from build123d import *

# Parameters (mm, degrees)
SALIENTE_EXTRUIR1_DEPTH = 6
CROQUIS2_W              = 10
CROQUIS2_H              = 6
CROQUIS2_W_2            = 6
CROQUIS2_H_2            = 10
CORTAR_EXTRUIR1_DEPTH   = 10


with BuildPart() as part:
    # Croquis1 → Saliente-Extruir1 (new body)
    with BuildSketch(Plane.XY):
        with BuildLine():
            ThreePointArc((40.600971411, -36.999917491), (17.069259083, -64.251458669), (-0.057755376, -95.922476295))
            ThreePointArc((-0.057755376, -95.922476295), (122.116838757, -322.352188967), (320.78926855, -158.870349387))
            ThreePointArc((320.78926855, -158.870349387), (317.672636714, -126.79639101), (308.439349644, -95.922476295))
            ThreePointArc((308.439349644, -95.922476295), (291.312335185, -64.251458669), (267.780622857, -36.999917491))
            ThreePointArc((267.780622857, -36.999917491), (154.190797134, 7.728122029), (40.600971411, -36.999917491))
        make_face()
        with BuildLine():
            ThreePointArc((50.939396199, -50.062499464), (51.321581101, -49.701102835), (51.705030941, -49.341048614))
            ThreePointArc((51.705030941, -49.341048614), (213.886421224, -21.26063874), (304.190797134, -158.870349387))
            ThreePointArc((304.190797134, -158.870349387), (94.978087942, -296.688545102), (50.939396199, -50.062499464))
        make_face(mode=Mode.SUBTRACT)
    extrude(amount=SALIENTE_EXTRUIR1_DEPTH)

    # Croquis2 → Cortar-Extruir1 (cut)
    with BuildSketch(Plane.XY.offset(6)):
        Polygon((139.190797134, -3.571113679), (149.190797134, -3.571113679), (149.190797134, -0.571113679), (149.190797134, 2.428886321), (139.190797134, 2.428886321), align=None)
        with Locations((164.190797134, -0.571113679)):
            Rectangle(CROQUIS2_W, CROQUIS2_H)
        with Locations((312.490032842, -148.870349387)):
            Rectangle(CROQUIS2_W_2, CROQUIS2_H_2)
        Polygon((312.490032842, -163.870349387), (315.490032842, -163.870349387), (315.490032842, -173.870349387), (309.490032842, -173.870349387), (309.490032842, -163.870349387), align=None)
        with Locations((164.190797134, -317.169585095)):
            Rectangle(CROQUIS2_W, CROQUIS2_H)
        Polygon((149.190797134, -317.169585095), (149.190797134, -314.169585095), (139.190797134, -314.169585095), (139.190797134, -320.169585095), (149.190797134, -320.169585095), align=None)
        with Locations((-4.108438574, -148.870349387)):
            Rectangle(CROQUIS2_W_2, CROQUIS2_H_2)
        Polygon((-7.108438574, -173.870349387), (-7.108438574, -163.870349387), (-4.108438574, -163.870349387), (-1.108438574, -163.870349387), (-1.108438574, -173.870349387), align=None)
        with BuildLine():
            ThreePointArc((40.806765207, -45.48631746), (40.806765207, -48.385455263), (43.705903009, -48.385455263))
            Line((43.705903009, -48.385455263), (40.806765207, -45.48631746))
        make_face()
        with BuildLine():
            Line((40.806765207, -45.48631746), (43.705903009, -48.385455263))
            ThreePointArc((43.705903009, -48.385455263), (44.15028715, -47.720387398), (44.306334108, -46.935886361))
            ThreePointArc((44.306334108, -46.935886361), (43.040835144, -45.04193332), (40.806765207, -45.48631746))
        make_face()
        with BuildLine():
            ThreePointArc((267.574829061, -45.48631746), (264.675691258, -45.48631746), (264.675691258, -48.385455263))
            Line((264.675691258, -48.385455263), (267.574829061, -45.48631746))
        make_face()
        with BuildLine():
            Line((267.574829061, -45.48631746), (264.675691258, -48.385455263))
            ThreePointArc((264.675691258, -48.385455263), (266.909761196, -48.829839403), (268.17526016, -46.935886361))
            ThreePointArc((268.17526016, -46.935886361), (268.019213202, -46.151385325), (267.574829061, -45.48631746))
        make_face()
        with BuildLine():
            ThreePointArc((268.17526016, -270.804812413), (266.909761196, -268.910859371), (264.675691258, -269.355243512))
            Line((264.675691258, -269.355243512), (267.574829061, -272.254381314))
            ThreePointArc((267.574829061, -272.254381314), (268.019213202, -271.589313449), (268.17526016, -270.804812413))
        make_face()
        with BuildLine():
            Line((267.574829061, -272.254381314), (264.675691258, -269.355243512))
            ThreePointArc((264.675691258, -269.355243512), (264.675691258, -272.254381314), (267.574829061, -272.254381314))
        make_face()
        with BuildLine():
            ThreePointArc((44.306334108, -270.804812413), (44.15028715, -270.020311377), (43.705903009, -269.355243512))
            Line((43.705903009, -269.355243512), (40.806765207, -272.254381314))
            ThreePointArc((40.806765207, -272.254381314), (43.040835144, -272.698765455), (44.306334108, -270.804812413))
        make_face()
        with BuildLine():
            Line((40.806765207, -272.254381314), (43.705903009, -269.355243512))
            ThreePointArc((43.705903009, -269.355243512), (40.806765207, -269.355243512), (40.806765207, -272.254381314))
        make_face()
    extrude(amount=-CORTAR_EXTRUIR1_DEPTH, mode=Mode.SUBTRACT)


solid = part.part
Verification items for the finished model (mm, model axes). Give positions to 0.01 mm unless a question says otherwise; leave off trailing zeros. Loops run counter-clockwise (first coordinate to the right, second up) from the corner with the lowest first, then second, coordinate; pieces in that order, holes last.
1) Depth check by flat-ended pin: pin 1 Ø1.5 at (x, y) = (69.5, -281) entering from -Z; pin 2 Ø1.8 at (x, z) = (165.5, 2.5) entering from +Y; pin 3 Ø1 at (y, z) = (-279, 4.5) entering from -X; pin 4 Ø3 at (x, z) = (73, 4.5) entering from +Y. Enter the tip coordinate at first touch or a pass-through.
2) Sectioned sample at B-B, the plane y = -204. Enter the section's corners in (x, z), then the cut area to 3 significant figures.
3) Sectioned sample at A-A, the plane x = 292. Enter the section's corners in (y, z), then the cut area to 3 significant figures.
4) Sectioned sample at C-C, the plane z = 4.2. Count the separate pieces of the cut face and the enclosed holes in it, then the cut area to 3 significant figures.
5) Thickness scan on line 1 along Y through (x, z) = (267.5, 1.6); line 2 along X through (y, z) = (-170.5, 2.65); line 3 along X through (y, z) = (-165.5, 3.85). Record the ranges inside material, lowest first.
Answers:
1. pin 1: passes through
1. pin 2: stops at y = 7.4
1. pin 3: stops at x = 38.24
1. pin 4: stops at y = -12.57
2. outline: (-6.18, 0) - (11.14, 0) - (11.14, 6) - (-6.18, 6) - close; (297.24, 0) - (314.56, 0) - (314.56, 6) - (297.24, 6) - close
2. area: 208 mm2
3. outline: (-252.48, 0) - (-218.1, 0) - (-218.1, 6) - (-252.48, 6) - close; (-99.64, 0) - (-65.26, 0) - (-65.26, 6) - (-99.64, 6) - close
3. area: 413 mm2
4. separate pieces: 1
4. enclosed holes: 13
4. area: 16,000 mm2
5. line 1: y = -281 to -272.33, -269.28 to -257.16, -60.58 to -48.46, -45.42 to -36.74
5. line 2: x = -12 to -7.11, -1.11 to 4.64, 303.74 to 309.49, 315.49 to 320.38
5. line 3: x = -12.28 to -7.11, -1.11 to 4.34, 304.04 to 309.49, 315.49 to 320.66
